For this review, take the finished solid that the model builds, in its own axes (mm). A direction names the side the tool comes from. Round coordinates to 2 decimals unless told otherwise and drop trailing zeros. Order: outer loops, then holes, each group sorted by start corner. A loop starts at its lowest first (then second) coordinate and runs counter-clockwise, first axis right, second up. Notation, with made-up numbers: (78.25, 28.25) -> (86.25, 28.25) arc R16 cw to (86.25, 57.25) -> close; hole circle Ø3 at (-39, -9). An arc over 180 degrees is marked (long way). Answer in a Markdown table with one row per item.
Autodesk Inventor part; units mm, degrees
ref_plane "YZ Plane" through (0, 0, 0) normal (1, 0, 0) x (0, 1, 0)
ref_plane "XZ Plane" through (0, 0, 0) normal (0, 1, 0) x (-1, 0, 0)
ref_plane "XY Plane" through (0, 0, 0) normal (0, 0, 1) x (1, 0, 0)
sketch "Sketch1" plane through (0, 0, 0) normal (0, 1, 0) x (-1, 0, 0)
  line L0 (0, 0) -> (-50, 0)
  line L1 (-50, 0) -> (-50, -130)
  line L2 (-50, -130) -> (0, -130)
  line L3 (0, -130) -> (0, 0)
  dimension "d0" = 130
  dimension "d1" = 50
extrude "Base" add sketch "Sketch1" along normal blind 3
sketch "Sketch2" plane through (0, 3, 0) normal (0, 1, 0) x (1, 0, 0)
  line L0 (0, 0) -> (50, 0)
  line L1 (50, 130) -> (0, 130)
  line L2 (0, 0) -> (3, 0)
  line L3 (3, 130) -> (0, 130)
  line L4 (0, 130) -> (0, 0)
  line L5 (0, 130) -> (0, 0)
  line L6 (0, 0) -> (3, 0)
  line L7 (3, 0) -> (3, 20)
  line L8 (3, 20) -> (0, 20)
  line L9 (0, 20) -> (0, 0)
  line L10 (0, 130) -> (3, 130)
  line L11 (3, 130) -> (3, 110)
  line L12 (3, 110) -> (0, 110)
  line L13 (0, 110) -> (0, 130)
  line L14 (0, 40) -> (3, 40)
  line L15 (3, 40) -> (3, 90)
  line L16 (3, 90) -> (0, 90)
  line L17 (0, 90) -> (0, 40)
  line L18 (25, 0) -> (25, 130) construction
  line L19 (50, 0) -> (47, 0)
  line L20 (47, 130) -> (50, 130)
  line L21 (50, 130) -> (50, 0)
  line L22 (50, 130) -> (50, 0)
  line L23 (50, 0) -> (47, 0)
  line L24 (47, 0) -> (47, 20)
  line L25 (47, 20) -> (50, 20)
  line L26 (50, 20) -> (50, 0)
  line L27 (50, 130) -> (47, 130)
  line L28 (47, 130) -> (47, 110)
  line L29 (47, 110) -> (50, 110)
  line L30 (50, 110) -> (50, 130)
  line L31 (50, 40) -> (47, 40)
  line L32 (47, 40) -> (47, 90)
  line L33 (47, 90) -> (50, 90)
  line L34 (50, 90) -> (50, 40)
  line L35 (15, 0) -> (35, 0)
  line L36 (35, 0) -> (35, 3)
  line L37 (35, 3) -> (15, 3)
  line L38 (15, 3) -> (15, 0)
  line L39 (0, 65) -> (50, 65) construction
  line L40 (50, 0) -> (50, 130)
  line L41 (35, 130) -> (35, 127)
  line L42 (35, 127) -> (15, 127)
  line L43 (15, 127) -> (15, 130)
  point P0 (0, 20)
  point P1 (0, 110)
  point P2 (0, 130)
  point P3 (0, 90)
  point P4 (0, 40)
  point P5 (15, 130)
  dimension "d10" = 20
  dimension "d11" = 20
  dimension "d12" = 20
  dimension "d13" = 20
  dimension "d14" = 50
  dimension "d15" = 3
  dimension "VerticalTab" = 20
  dimension "d19" = 10
  dimension "d20" = 3
extrude "Tabs" cut sketch "Sketch2" against normal through all contours L4 L8 L7 L0 | L38 L37 L36 L0 | L4 L16 L15 L14 | L24 L25 L21 L0 | L4 L1 L11 L12 | L31 L32 L33 L21 | L1 L41 L42 L43 | L29 L28 L1 L21
equation "\"d0\" = Length"
equation "\"d2\" = Thickness"
equation "\"d10\" = LengthTabOffset"
equation "\"d11\" = LengthTabOffset"
equation "\"d12\" = BaseTabWidth"
equation "\"d13\" = BaseTabWidth"
equation "\"d15\" = Thickness"
equation "\"d19\" = 0.5 * VerticalTab"
equation "\"d20\" = d15"
properties part number "LongSide"
Q1. Tool access review of faces 5 (the face through (48, 2, -90)), 6 (the face through (3, 2, -120)), 7 (the face through (2, 2, -20)), 8 (the face through (3, 2, -65)): name each direction out of +Z, -Z, +X, -X, +Y, -Y from which nothing blocks a thin tool from reaching the whole face with its end or side.
Answer key:
| item | result |
|---|---|
| face 5 | +X, +Y, -Y |
| face 6 | -Z, -X, +Y, -Y |
| face 7 | +Z, -X, +Y, -Y |
| face 8 | -X, +Y, -Y |
Q2. Clearance check with flat-ended pins moving along their axes: pin 1 Ø12 at (x, z) = (30, -115) entering from -Y; pin 2 Ø1.5 at (y, z) = (1.5, -123) entering from +X; pin 3 Ø1.5 at (y, z) = (1.5, -7) entering from -X; pin 4 Ø0.9 at (x, y) = (1.5, 1) entering from +Z. State where each tip first meets the part, or that it passes through.
Answer key:
| item | result |
|---|---|
| pin 1 | stops at y = 0 |
| pin 2 | stops at x = 47 |
| pin 3 | stops at x = 3 |
| pin 4 | stops at z = -20 |
Q3. Take a section at A-A, the plane y = 0.5. Write out the cut boundary in (x, z), then the cut area to 3 significant figures.
Answer key:
| item | result |
|---|---|
| outline | (0, -110) -> (3, -110) -> (3, -130) -> (15, -130) -> (15, -127) -> (35, -127) -> (35, -130) -> (47, -130) -> (47, -110) -> (50, -110) -> (50, -90) -> (47, -90) -> (47, -40) -> (50, -40) -> (50, -20) -> (47, -20) -> (47, 0) -> (35, 0) -> (35, -3) -> (15, -3) -> (15, 0) -> (3, 0) -> (3, -20) -> (0, -20) -> (0, -40) -> (3, -40) -> (3, -90) -> (0, -90) -> close |
| area | 5,840 mm^2 |
Q4. The part is to be moulded in two halves that separate along X. For faces 1 (the face through (1, 2, -40)), 2 (the face through (35, 2, -129)), 3 (the face through (0, 1, -100)), 4 (the face through (25, 2, -3)), say which applies: +X half, -X half, draft (parallel to the pull), parting line (faces both ways), or undercut.
Answer key:
| item | result |
|---|---|
| face 1 | draft |
| face 2 | undercut |
| face 3 | -X half |
| face 4 | undercut |
Q5. Take a section at C-C, the plane z = -47. Write out the cut boundary in (x, y), then the cut area to 3 significant figures.
Answer key:
| item | result |
|---|---|
| outline | (3, 0) -> (47, 0) -> (47, 3) -> (3, 3) -> close |
| area | 132 mm^2 |
Q6. Take a section at B-B, the plane x = 17. Write out the cut boundary in (y, z), then the cut area to 3 significant figures.
Answer key:
| item | result |
|---|---|
| outline | (0, -127) -> (3, -127) -> (3, -3) -> (0, -3) -> close |
| area | 372 mm^2 |
Q7. To check wall thickness, follow probe 1 along X at (y, z) = (0.15, -9.5); probe 2 along Z at (x, y) = (19, 1.4). State the ranges of each line that lie inside material, in increasing order.
Answer key:
| item | result |
|---|---|
| probe 1 | x = 3 to 47 |
| probe 2 | z = -127 to -3 |
